Input: part model. Units: mm. Frame: model coordinates. A direction names the side the tool comes from. Coordinates: 2 decimals unless noted, no trailing zeros. Loops run counter-clockwise (first coordinate to the right, second up) from the corner with the lowest first, then second, coordinate; pieces in that order, holes last.
```python
from build123d import *

# Parameters (mm, degrees)
PAD003_DEPTH = 1
PAD004_DEPTH = 1
PAD_DEPTH    = 25


with BuildPart() as pad003:
    # Sketch001 → Pad003 (new body)
    with BuildSketch(Plane.XY.offset(32)):
        with BuildLine():
            Line((-5.8767, 4.245809), (-8.700179, 4.930201))
            ThreePointArc((0, 10), (-5.034779, 8.640081), (-8.700179, 4.930201))
            Line((0, 10), (4.98503, 15))
            Line((10, 15), (4.98503, 15))
            Line((10, -15), (10, 15))
            Line((4.98503, -15), (10, -15))
            Line((0, -10), (4.98503, -15))
            Line((0, -7.25), (0, -10))
            ThreePointArc((0, -7.25), (6.455409, 3.300029), (-5.8767, 4.245809))
        make_face()
    extrude(amount=PAD003_DEPTH)


with BuildPart() as pad004:
    # Sketch002 → Pad004 (new body)
    with BuildSketch(Plane.XY.offset(48)):
        with BuildLine():
            Line((-5.8767, 4.245809), (-8.700179, 4.930201))
            ThreePointArc((0, 10), (-5.034779, 8.640081), (-8.700179, 4.930201))
            Line((0, 10), (4.98503, 15))
            Line((10, 15), (4.98503, 15))
            Line((10, -15), (10, 15))
            Line((4.98503, -15), (10, -15))
            Line((0, -10), (4.98503, -15))
            Line((0, -7.25), (0, -10))
            ThreePointArc((0, -7.25), (6.455409, 3.300029), (-5.8767, 4.245809))
        make_face()
    extrude(amount=PAD004_DEPTH)


with BuildPart() as obj1:
    # Sketch → Pad (new body)
    with BuildSketch(Plane.XY.offset(28)):
        with BuildLine():
            Line((-6.124049, 4.274369), (-8.700179, 4.930201))
            ThreePointArc((0, 10), (-5.034779, 8.640081), (-8.700179, 4.930201))
            Line((0, 10), (4.98503, 15))
            Line((10, 15), (4.98503, 15))
            Line((10, -15), (10, 15))
            Line((4.98503, -15), (10, -15))
            Line((0, -9.952784), (4.98503, -15))
            Line((0, -7.468213), (0, -9.952784))
            ThreePointArc((0, -7.468213), (6.621786, 3.453426), (-6.124049, 4.274369))
        make_face()
    extrude(amount=PAD_DEPTH)

    # Fusion: union Pad003, Pad004
    add(pad003.part)
    add(pad004.part)


solid = obj1.part
```
Item 1: Mould query, pull axis Z, two halves, no side actions, for faces 1 (the face through (8, 1, 28)), 2 (the face through (8, 15, 40)), 3 (the face through (2.458, -12.441, 40.395)). Classes: +Z half, -Z half, draft (parallel to the pull), parting line (faces both ways), or undercut.
Result:
face 1: -Z half
face 2: draft
face 3: undercut
Item 2: Reachability of faces 4 (the face through (2.458, -12.441, 29.972)), 5 (the face through (6.55, 3.11, 32.49)), 6 (the face through (0, -9, 40)) from +Z, -Z, +X, -X, +Y, -Y: full face, straight path, thin tool, end or side. Return the list, or none.
Result:
face 4: -Z, -X, -Y
face 5: +Z, -Z
face 6: +Z, -Z, -X, -Y
Item 3: Section query B-B (y = 0). Output: boundary loops of the cut face in (x, z), then the cut area to 3 significant figures.
Result:
outline: (7.25, 32) - (7.47, 32) - (7.47, 28) - (10, 28) - (10, 53) - (7.47, 53) - (7.47, 49) - (7.25, 49) - (7.25, 48) - (7.47, 48) - (7.47, 33) - (7.25, 33) - close
area: 63.7 mm2
Item 4: Contact query for flat-ended pins moving along their axis: P1, Ø2, axis at x = -6.5, z = 36.5, coming from the +Y side; P2, Ø3, axis at x = -6.5, z = 38.5, coming from the -Y side; P3, Ø6, axis at y = -1.5, z = 37.5, coming from the -X side. Output: stop coordinate, or through.
Result:
P1: stops at y = 8.35
P2: stops at y = 4.27
P3: stops at x = 5.96
Item 5: Section query A-A (z = 34.75). Output: boundary loops of the cut face in (x, y), then the cut area to 3 significant figures.
Result:
outline: (-8.7, 4.93) - (-6.12, 4.27) arc R7.47 cw (long way) to (0, -7.47) - (0, -9.95) - (4.99, -15) - (10, -15) - (10, 15) - (4.99, 15) - (0, 10) arc R10 ccw to start
area: 210 mm2
Item 6: Section query D-D (x = -2.5). Output: boundary loops of the cut face in (y, z).
Result:
outline: (6.81, 32) - (7.04, 32) - (7.04, 28) - (9.68, 28) - (9.68, 53) - (7.04, 53) - (7.04, 49) - (6.81, 49) - (6.81, 48) - (7.04, 48) - (7.04, 33) - (6.81, 33) - close
Item 7: Line query: L1, parallel to X at y = 0, z = 32.45; L2, parallel to X at y = 5.25, z = 41.25; L3, parallel to Y at x = 5, z = 30. Output: solid intervals per line, ascending.
Result:
L1: x = 7.25 to 10
L2: x = -8.51 to -5.31, 5.31 to 10
L3: y = -15 to -5.55, 5.55 to 15
